Verification items for this drawing (mm, ordinates from the low corner). Round coordinates to 2 decimals unless told otherwise and drop trailing zeros. Write each loop counter-clockwise with the first axis right and the second up, starting at its lowest first coordinate (ties: lowest second). Pieces come first, ordered by that corner, then holes.
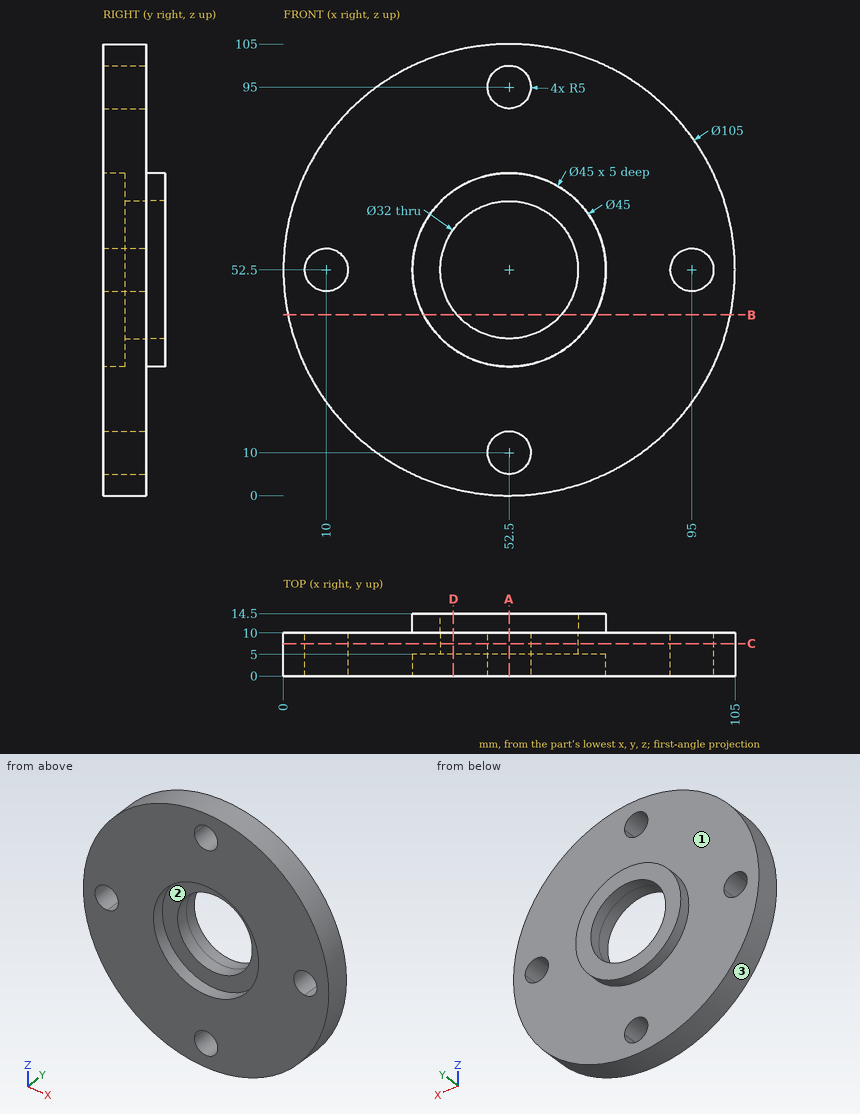
1. Release check for a two-part mould opening along X. For the marked faces 1, 2 and 3 record: +X half, -X half, draft (parallel to the pull), parting line (faces both ways), or undercut.
2. Section check C-C (y = 7.5). Record the cut outline in (x, z).
3. Section check D-D (x = 39.5). Record the cut outline in (y, z).
4. Section check A-A (x = 52.5). Record the cut outline in (y, z), plus the area to 4 significant figures.
5. Scan lines: line 1 along Z through (x, y) = (52.5, 2.65); line 2 along X through (y, z) = (4.5, 50.5); line 3 along Y through (x, z) = (87, 45). Record each from-to range of solid material in increasing order.
6. Depth check by flat-ended pin: pin 1 Ø1 at (x, y) = (93, 2) entering from -Z; pin 2 Ø4 at (y, z) = (10.5, 40.5) entering from -X; pin 3 Ø13.5 at (x, z) = (47, 49) entering from -Y; pin 4 Ø5 at (x, y) = (13, 7) entering from -Z. Enter the tip coordinate at first touch or a pass-through.
7. Section check B-B (z = 42). Record the cut outline in (x, y).
Results below:
1. face 1: draft
1. face 2: undercut
1. face 3: parting line
2. outline: circle Ø105 at (52.5, 52.5); hole circle Ø10 at (10, 52.5); hole circle Ø32 at (52.5, 52.5); hole circle Ø10 at (52.5, 10); hole circle Ø10 at (52.5, 95); hole circle Ø10 at (95, 52.5)
3. outline: (0, 1.63) - (10, 1.63) - (10, 34.14) - (14.5, 34.14) - (14.5, 43.17) - (5, 43.17) - (5, 34.14) - (0, 34.14) - close; (0, 70.86) - (5, 70.86) - (5, 61.83) - (14.5, 61.83) - (14.5, 70.86) - (10, 70.86) - (10, 103.37) - (0, 103.37) - close
4. outline: (0, 0) - (10, 0) - (10, 5) - (0, 5) - close; (0, 15) - (10, 15) - (10, 30) - (14.5, 30) - (14.5, 36.5) - (5, 36.5) - (5, 30) - (0, 30) - close; (0, 75) - (5, 75) - (5, 68.5) - (14.5, 68.5) - (14.5, 75) - (10, 75) - (10, 90) - (0, 90) - close; (0, 100) - (10, 100) - (10, 105) - (0, 105) - close
4. area: 523.5 mm2
5. line 1: z = 0 to 5, 15 to 30, 75 to 90, 100 to 105
5. line 2: x = 0.04 to 5.42, 14.58 to 30.09, 74.91 to 90.42, 99.58 to 104.96
5. line 3: y = 0 to 10
6. pin 1: stops at z = 18.5
6. pin 2: stops at x = 0.97
6. pin 3: passes through
6. pin 4: stops at z = 15.25
7. outline: (1.06, 0) - (32.6, 0) - (32.6, 5) - (40.43, 5) - (40.43, 14.5) - (32.6, 14.5) - (32.6, 10) - (1.06, 10) - close; (64.57, 5) - (72.4, 5) - (72.4, 0) - (103.94, 0) - (103.94, 10) - (72.4, 10) - (72.4, 14.5) - (64.57, 14.5) - close
